Geometry check sheet. Reference: the model listing, model coordinates, mm. A direction names the side the tool comes from. Round coordinates to 2 decimals unless told otherwise and drop trailing zeros. Order: outer loops, then holes, each group sorted by start corner. A loop starts at its lowest first (then second) coordinate and runs counter-clockwise, first axis right, second up. Notation, with made-up numbers: (80.25, 16) - (89.25, 16) arc R33 ccw to (89.25, 49) - close; hole circle Ø8 at (-2, 31). An arc over 180 degrees is marked (long way). Write each question's results on one line, items separated by ' | '.
```python
from build123d import *

# Parameters (mm, degrees)
EXTRUDE_1_DEPTH     = 6
SKETCH_2_R          = 1.1
CUT_EXTRUDE_1_DEPTH = 19.661457607
CUT_EXTRUDE_START   = 4
SKETCH_3_R          = 2.05
CUT_EXTRUDE_2_DEPTH = 15.661457773


with BuildPart() as part:
    # Эскиз1 → Бобышка-Вытянуть1 (new body)
    with BuildSketch(Plane(origin=(0, 0, 0), x_dir=(1, 0, 0), z_dir=(0, 1, 0))):
        with BuildLine():
            ThreePointArc((12.5, 0), (9.013878189, 8.660254038), (0.5, 12.489995997))
            Line((0.5, 12.489995997), (0.5, 3.160696126))
            ThreePointArc((0.5, 3.160696126), (2.433105012, 2.078460969), (3.2, 0))
            ThreePointArc((3.2, 0), (2.433105012, -2.078460969), (0.5, -3.160696126))
            Line((0.5, -3.160696126), (0.5, -12.489995997))
            ThreePointArc((0.5, -12.489995997), (9.013878189, -8.660254038), (12.5, 0))
        make_face()
    extrude(amount=EXTRUDE_1_DEPTH)

    # Эскиз2 → Вырез-Вытянуть1 (cut, through all)
    with BuildSketch(Plane(origin=(0, 0, 0), x_dir=(0, 0, -1), z_dir=(1, 0, 0))):
        with Locations(Location((7.825346061, 3, 0), (0, 0, 180))):
            Circle(SKETCH_2_R)
        with Locations(Location((-7.825346061, 3, 0), (0, 0, 180))):
            Circle(SKETCH_2_R)
    extrude(amount=CUT_EXTRUDE_1_DEPTH, mode=Mode.SUBTRACT)

    # Эскиз3 → Вырез-Вытянуть2 (cut, through all)
    with BuildSketch(Plane(origin=(0, 0, 0), x_dir=(0, 0, -1), z_dir=(1, 0, 0)).offset(CUT_EXTRUDE_START)):
        with Locations(Location((7.825346061, 3, 0), (0, 0, 180))):
            Circle(SKETCH_3_R)
        Polygon((-9.008914113, 0.95), (-6.641778009, 0.95), (-5.458209958, 3), (-6.641778009, 5.05), (-9.008914113, 5.05), (-10.192482165, 3), align=None)
    extrude(amount=CUT_EXTRUDE_2_DEPTH, mode=Mode.SUBTRACT)


solid = part.part
```
(1) Section check D-D (y = 2.25). Record the cut outline in (x, z), then the cut area to 3 significant figures.
Answers follow:
outline: (0.5, -12.49) arc R12.5 ccw to (7.84, -9.73) - (4, -9.73) - (4, -8.63) - (0.5, -8.63) - close; (0.5, -7.02) - (4, -7.02) - (4, -5.92) - (11.01, -5.92) arc R12.5 ccw to (11.02, 5.89) - (4, 5.89) - (4, 7.02) - (0.5, 7.02) - (0.5, 3.16) arc R3.2 cw to (0.5, -3.16) - close; (0.5, 8.63) - (4, 8.63) - (4, 9.76) - (7.81, 9.76) arc R12.5 ccw to (0.5, 12.49) - close | area: 165 mm²
(2) Depth check by flat-ended pin: pin 1 Ø2 at (y, z) = (3, -7.83) entering from -X (3 decimals); pin 2 Ø1.5 at (y, z) = (2.5, 6) entering from +X; pin 3 Ø3 at (x, y) = (11, 1) entering from +Z; pin 4 Ø3.5 at (y, z) = (3.5, -8.5) entering from +X. Enter the tip coordinate at first touch or a pass-through.
Answers follow:
pin 1: through | pin 2: x = 11.34 | pin 3: z = 8.12 | pin 4: x = 9.86
(3) Section check C-C (z = 8.5). Record the cut outline in (x, y).
Answers follow:
outline: (0.5, 0) - (9.17, 0) - (9.17, 0.95) - (4, 0.95) - (4, 2.13) - (0.5, 2.13) - close; (0.5, 3.87) - (4, 3.87) - (4, 5.05) - (9.17, 5.05) - (9.17, 6) - (0.5, 6) - close
(4) Material ranges on line 1 (Z direction, x = 6.25, y = 3.75); line 2 (Z direction, x = 4.25, y = 3.75); line 3 (Z direction, x = 2, y = 4.5), recorded low to high.
Answers follow:
line 1: -10.83 to -9.73, -5.92 to 5.89, 9.76 to 10.83 | line 2: -11.76 to -9.73, -5.92 to 5.89, 9.76 to 11.76 | line 3: -12.34 to -2.5, 2.5 to 12.34
(5) Section check A-A (x = 2.75). Record the cut outline in (y, z), then the cut area to 3 significant figures.
Answers follow:
outline: (0, -12.19) - (6, -12.19) - (6, -1.64) - (0, -1.64) - close; (0, 1.64) - (6, 1.64) - (6, 12.19) - (0, 12.19) - close; hole circle Ø2.2 at (3, -7.83); hole circle Ø2.2 at (3, 7.83) | area: 119 mm²
(6) Draft check along Z on faces 3 (the face through (0.5, 2, 7)), 4 (the face through (4, 2, 7)), 5 (the face through (7.57, 4.01, 6.04)). Enter one of: released by +Z, released by -Z, zero draft, split by the parting line, or undercut.
Answers follow:
face 3: zero draft | face 4: undercut | face 5: undercut
(7) Section check B-B (y = 5.5). Record the cut outline in (x, z), then the cut area to 3 significant figures.
Answers follow:
outline: (0.5, -12.49) arc R12.5 ccw to (0.5, 12.49) - (0.5, 3.16) arc R3.2 cw to (0.5, -3.16) - close | area: 220 mm²
(8) Access from +Z, -Z, +X, -X, +Y, -Y to the whole of each face (thin tool, end or side, straight path). Record for faces 1 (the face through (2.226, 2.67, 8.875)), 2 (the face through (6.71, 2.38, -5.87)).
Answers follow:
face 1: +X, -X | face 2: +X
